```python
from build123d import *

# Parameters (mm, degrees)
AUFSATZ_LINEAR_AUSTRAGEN1_DEPTH = 2
VERRUNDUNG6_R                   = 5
VERRUNDUNG7_R                   = 10
SKIZZE4_R                       = 3
SCHNITT_LINEAR_AUSTRAGEN1_DEPTH = 2


with BuildPart() as part:
    # Skizze2 → Aufsatz-Linear austragen1 (new body)
    with BuildSketch(Plane(origin=(0, 0, 0), x_dir=(0, 0, -1), z_dir=(1, 0, 0))):
        Polygon((0, 0), (-86.9, 0), (-86.9, 43), (-80, 47), (-80, 106.8), (-28.6, 106.8), (-28.6, 51.396087758), (-17, 51.396087758), (-17, 39.8), (0, 39.8), (0, 33.4), (-10.333924714, 27.3), (-15, 27), (-15, 23.4), (0, 23.4), align=None)
    extrude(amount=-AUFSATZ_LINEAR_AUSTRAGEN1_DEPTH)

    # Verrundung6
    verrundung6_edges = [part.edges().sort_by_distance(p)[0] for p in [
        (-1, 0, 0),
        (-1, 106.8, 80),
        (-1, 106.8, 28.6),
        (-1, 39.8, 0),
    ]]
    fillet(verrundung6_edges, radius=VERRUNDUNG6_R)

    # Verrundung7
    verrundung7_edges = [part.edges().sort_by_distance(p)[0] for p in [
        (-1, 27.3, 10.333924714),
    ]]
    fillet(verrundung7_edges, radius=VERRUNDUNG7_R)

    # Skizze4 → Schnitt-Linear austragen1 (cut)
    with BuildSketch(Plane(origin=(0, 0, 0), x_dir=(0, 0, -1), z_dir=(1, 0, 0))):
        with Locations((-65, 25)):
            Circle(SKIZZE4_R)
    extrude(amount=-SCHNITT_LINEAR_AUSTRAGEN1_DEPTH, mode=Mode.SUBTRACT)


solid = part.part
```
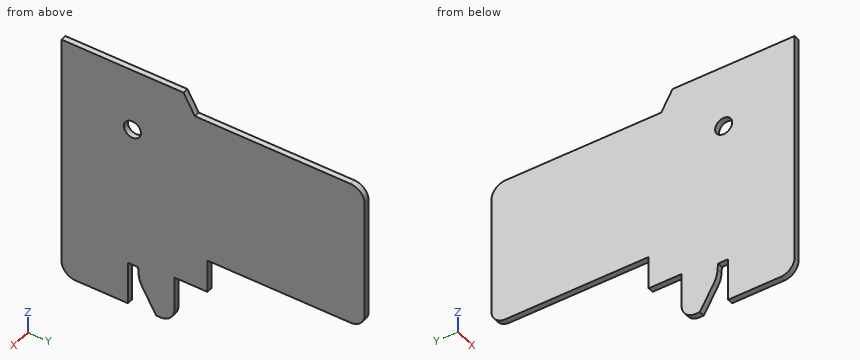
CAD build for the part. Positions are in the model's coordinates, mm. Round coordinates to 2 decimals unless told otherwise and drop trailing zeros. Order: outer loops, then holes, each group sorted by start corner. A loop starts at its lowest first (then second) coordinate and runs counter-clockwise, first axis right, second up.
Item 1: Saw through at B-B on x = -1.15. Write the cut outline in (y, z).
Item 2: Probe line 1 along Y through (x, z) = (-0.35, 65); line 2 along Z through (x, y) = (-1.6, 100); line 3 along Y through (x, z) = (-0.65, 28.5). List the from-to ranges inside material, lowest first.
Item 3: Saw through at D-D on y = 45. Write the cut outline in (x, z).
Item 4: Saw through at A-A on z = 65. Write the cut outline in (x, y), then the cut area to 3 significant figures.
Item 5: Pin check, flat tips, straight feed: pin 1 (0.6 mm diameter, centred on x = -0.5, y = 25, fed in from -Z); pin 2 (3 mm diameter, centred on y = 41.5, z = 16, fed in from -X); pin 3 (1 mm diameter, centred on x = -1.5, y = 75.5, fed in from +Z); pin 4 (1 mm diameter, centred on x = -1.5, z = 29.5, fed in from +Y). Stop position of each tip, or through.
Item 6: Saw through at C-C on y = 25. Write the cut outline in (x, z).
Reported:
1. outline: (0, 5) arc R5 ccw to (5, 0) - (23.4, 0) - (23.4, 15) - (27, 15) - (27.15, 12.72) arc R10 ccw to (28.51, 8.28) - (33.4, 0) - (34.8, 0) arc R5 ccw to (39.8, 5) - (39.8, 17) - (51.4, 17) - (51.4, 28.6) - (101.8, 28.6) arc R5 ccw to (106.8, 33.6) - (106.8, 75) arc R5 ccw to (101.8, 80) - (47, 80) - (43, 86.9) - (0, 86.9) - close; hole circle Ø6 at (25, 65)
2. line 1: y = 0 to 22, 28 to 106.8
2. line 2: z = 28.6 to 80
2. line 3: y = 0 to 51.4
3. outline: (-2, 17) - (0, 17) - (0, 83.45) - (-2, 83.45) - close
4. outline: (-2, 0) - (0, 0) - (0, 22) - (-2, 22) - close; (-2, 28) - (0, 28) - (0, 106.8) - (-2, 106.8) - close
4. area: 202 mm2
5. pin 1: stops at z = 15
5. pin 2: stops at x = -2
5. pin 3: stops at z = 80
5. pin 4: stops at y = 105.27
6. outline: (-2, 15) - (0, 15) - (0, 62) - (-2, 62) - close; (-2, 68) - (0, 68) - (0, 86.9) - (-2, 86.9) - close
